Part model, mm, in its own coordinate system. A direction names the side the tool comes from. Give positions to 0.01 mm unless a question says otherwise; leave off trailing zeros. Order: outer loops, then holes, each group sorted by start corner. A loop starts at its lowest first (then second) coordinate and runs counter-clockwise, first axis right, second up. Notation, with made-up numbers: (-7, 35) -> (37, 35) arc R12 ccw to (37, 39) -> close; hole circle Ø10 at (-18.5, 24.5). An arc over 180 degrees is marked (long way). Write item = value, one per line. Start each with the question number.
Item 1: Drill centre lines: line 1 along Z through (x, y) = (0, 0.25); line 2 along X through (y, z) = (-5, -0.05); line 3 along Y through (x, z) = (0, -0.05). Where is each one in solid material? Low to high.
Item 2: Band-saw the part on D-D on y = -0.75. Write the cut outline in (x, z).
Item 3: Tool access for faces 1 (the face through (0.429, 0.296, 1.933)), 2 (the face through (1, 0, 1)), 3 (the face through (1, 1, 0.35)): list every direction of +Z, -Z, +X, -X, +Y, -Y with a clear straight run to the whole face (end or side of a thin tool).
Item 4: Flat gauge pins, fed straight in: P1, Ø1, axis at y = 1, z = 1, coming from the +X side; P2, Ø1, axis at x = 1.5, z = -1, coming from the -Y side; P3, Ø0.5, axis at x = 1, y = 1, coming from the +Z side. Where does each tip first touch, or does it go through?
Item 5: Band-saw the part on A-A on y = 0.5. Write the cut outline in (x, z), plus the area to 3 significant figures.
Item 6: Pull direction Z, two halves, no side cores. Call faces 4 (the face through (-0.27, -2.96, 1.22)), 5 (the face through (-1, 1, 0.35)), 6 (the face through (0, -6, 0)): +Z half, -Z half, draft (parallel to the pull), parting line (faces both ways), or undercut.
Autodesk Inventor part; units mm, degrees
ref_plane "YZ Plane" through (0, 0, 0) normal (1, 0, 0) x (0, 1, 0)
ref_plane "XZ Plane" through (0, 0, 0) normal (0, 1, 0) x (-1, 0, 0)
ref_plane "XY Plane" through (0, 0, 0) normal (0, 0, 1) x (1, 0, 0)
sketch "Sketch1" plane through (0, 0, 0) normal (0, 1, 0) x (-1, 0, 0)
  circle A0 centre (0, 0) radius 1.98
  dimension "d0" = 3.96
extrude "Extrusion1" add sketch "Sketch1" along normal blind 1.6
sketch "Sketch2" plane through (0, 1.6, 0) normal (0, 1, 0) x (1, 0, 0)
  line L0 (-0.35, -0.35) -> (-1.25, -0.35)
  line L1 (-1.25, -0.35) -> (-1.25, 0.35)
  line L2 (-1.25, 0.35) -> (-0.35, 0.35)
  line L3 (-0.35, 0.35) -> (-0.35, 1.25)
  line L4 (-0.35, 1.25) -> (0.35, 1.25)
  line L5 (0.35, 1.25) -> (0.35, 0.35)
  line L6 (0.35, 0.35) -> (1.25, 0.35)
  line L7 (1.25, 0.35) -> (1.25, -0.35)
  line L8 (1.25, -0.35) -> (0.35, -0.35)
  line L9 (0.35, -1.25) -> (-0.35, -1.25)
  line L10 (-0.35, -1.25) -> (-0.35, -0.35)
  line L11 (0.35, -0.35) -> (0.35, -1.25)
  point P0 (0, 0)
  point P1 (0, -1.25)
  point P2 (0, 1.25)
  point P3 (-1.25, 0)
  point P4 (1.25, 0)
  dimension "d3" = 2.5
  dimension "d4" = 2.5
  dimension "d5" = 1.25
  dimension "d6" = 1.25
  dimension "d7" = 0.7
  dimension "d8" = 0.7
extrude "Extrusion2" cut sketch "Sketch2" against normal blind 2
fillet "Fillet1" radius 1 1 edges at (1.98, 1.6, 0)
sketch "Sketch3" plane through (0, 0, 0) normal (0, -1, 0) x (1, 0, 0)
  circle A0 centre (0, 0) radius 1.25
  dimension "d12" = 2.5
extrude "Extrusion3" add sketch "Sketch3" along normal blind 6
thread "Thread1"
equation "\"d4\" = d3"
equation "\"d8\" = d7"
properties part number "M4_8mm" material "Stainless Steel"
Values found:
q1.line_1 = -1.98 to -1.25, 1.25 to 1.98
q1.line_2 = -1.25 to 1.25
q1.line_3 = -6 to 0
q2.outline = circle Ø2.5 at (0, 0)
q3.face_1 = +Y, -Y
q3.face_2 = -Y
q3.face_3 = +Y
q4.P1 = 1.89
q4.P2 = 0
q4.P3 = 1.78
q5.outline = circle Ø3.96 at (0, 0); hole (-1.25, -0.35) -> (-0.35, -0.35) -> (-0.35, -1.25) -> (0.35, -1.25) -> (0.35, -0.35) -> (1.25, -0.35) -> (1.25, 0.35) -> (0.35, 0.35) -> (0.35, 1.25) -> (-0.35, 1.25) -> (-0.35, 0.35) -> (-1.25, 0.35) -> close
q5.area = 9.31 mm^2
q6.face_4 = parting line
q6.face_5 = undercut
q6.face_6 = draft
